```python
from build123d import *

# Parameters (mm, degrees)
SKETCH1_R                         = 60
BASE_BASE_DEPTH                   = 4
SIDE_START                        = -4
SIDE_CUTS_DEPTH                   = 4
SKETCH3_W                         = 5
SKETCH3_H                         = 13
TENDON_PASS_THROUGH_OPENING_DEPTH = 4
SKETCH4_R                         = 2.5
BASE_MOUNTING_HOLES_DEPTH         = 79.461200603
SKETCH5_W                         = 3
SKETCH5_H                         = 40
SKETCH5_W_2                       = 2.5
SKETCH5_H_2                       = 65
BOSS_EXTRUDE1_DEPTH               = 50
LPATTERN1_COUNT                   = 2
LPATTERN1_PITCH                   = 54
CUT_EXTRUDE1_REACH                = 138.279
SKETCH7_R                         = 3
CUT_EXTRUDE2_START                = -35
SKETCH9_R                         = 1
CUT_EXTRUDE2_DEPTH                = 35
LPATTERN2_COUNT                   = 2
LPATTERN2_PITCH                   = 96.6
FILLET1_R                         = 1
FILLET2_R                         = 1
SKETCH11_W                        = 12
SKETCH11_H                        = 6
CUT_EXTRUDE3_DEPTH                = 41
FILLET3_R                         = 1
FILLET4_R                         = 1
CUT_EXTRUDE4_REACH                = 104.781
SKETCH12_W                        = 20
SKETCH12_H                        = 8
FILLET5_R                         = 1


with BuildPart() as part:
    # Sketch1 → Base Base (new body)
    with BuildSketch(Plane(origin=(0, 0, 0), x_dir=(1, 0, 0), z_dir=(0, 1, 0))):
        with Locations(Location((0, 0, 0), (0, 0, 270))):
            Circle(SKETCH1_R)
    base_base = extrude(amount=BASE_BASE_DEPTH)

    # Sketch2 → Side Cuts (cut)
    with BuildSketch(Plane(origin=(0, 4, 0), x_dir=(1, 0, 0), z_dir=(0, 1, 0)).offset(SIDE_START)):
        with BuildLine():
            Line((-32.555183919, 50.4), (32.555183919, 50.4))
            ThreePointArc((32.555183919, 50.4), (0, 60), (-32.555183919, 50.4))
        make_face()
        with BuildLine():
            Line((-32.555183919, -50.4), (32.555183919, -50.4))
            ThreePointArc((32.555183919, -50.4), (0, -60), (-32.555183919, -50.4))
        make_face()
    extrude(amount=SIDE_CUTS_DEPTH, mode=Mode.SUBTRACT)

    # Sketch3 → Tendon Pass Through Opening (cut)
    with BuildSketch(Plane(origin=(0, 4, 0), x_dir=(1, 0, 0), z_dir=(0, 1, 0))):
        with Locations((32.5, 0)):
            Rectangle(SKETCH3_W, SKETCH3_H)
        with Locations((-32.5, 0)):
            Rectangle(SKETCH3_W, SKETCH3_H)
    extrude(amount=-TENDON_PASS_THROUGH_OPENING_DEPTH, mode=Mode.SUBTRACT)

    # Sketch4 → Base Mounting Holes (cut, through all)
    with BuildSketch(Plane(origin=(0, 4, 0), x_dir=(1, 0, 0), z_dir=(0, 1, 0))):
        with Locations(Location((32.5, 19, 0), (0, 0, 270))):
            Circle(SKETCH4_R)
        with Locations(Location((32.5, -19, 0), (0, 0, 90))):
            Circle(SKETCH4_R)
        with Locations(Location((-32.5, -19, 0), (0, 0, 270))):
            Circle(SKETCH4_R)
        with Locations(Location((-32.5, 19, 0), (0, 0, 90))):
            Circle(SKETCH4_R)
    extrude(amount=-BASE_MOUNTING_HOLES_DEPTH, mode=Mode.SUBTRACT)

    # Sketch5 → Boss-Extrude1 (add)
    with BuildSketch(Plane.XZ):
        with Locations((-48.3, -6)):
            Rectangle(SKETCH5_W, SKETCH5_H)
        with Locations((16.25, 11.5)):
            Rectangle(SKETCH5_W_2, SKETCH5_H_2)
        with Locations((48.3, -6)):
            Rectangle(SKETCH5_W, SKETCH5_H)
        with Locations((-16.25, 11.5)):
            Rectangle(SKETCH5_W_2, SKETCH5_H_2)
    extrude(amount=BOSS_EXTRUDE1_DEPTH)

    # LPattern1: Base Base ×2
    with Locations(*[(0, -i * LPATTERN1_PITCH, 0) for i in range(1, LPATTERN1_COUNT)]):
        add(base_base)

    # Sketch7 → Cut-Extrude1 (cut, up to next)
    with BuildSketch(Plane.ZY.offset(49.8), mode=Mode.PRIVATE) as cut_extrude1_sk1:
        with Locations((5.177676652, -18.760132428)):
            Circle(SKETCH7_R)
    cut_extrude1_tool1 = extrude(cut_extrude1_sk1.sketch, amount=-CUT_EXTRUDE1_REACH, mode=Mode.PRIVATE) & part.part
    # Sketch7 → Cut-Extrude1 (cut, up to next)
    with BuildSketch(Plane.ZY.offset(49.8), mode=Mode.PRIVATE) as cut_extrude1_sk2:
        with Locations((5.177676652, -42.760132428)):
            Circle(SKETCH7_R)
    cut_extrude1_tool2 = extrude(cut_extrude1_sk2.sketch, amount=-CUT_EXTRUDE1_REACH, mode=Mode.PRIVATE) & part.part
    cut_extrude1_1 = cut_extrude1_tool1.solids().sort_by_distance((-49.8, -18.760132, 5.177677))[0]
    add(cut_extrude1_1, mode=Mode.SUBTRACT)
    cut_extrude1_2 = cut_extrude1_tool2.solids().sort_by_distance((-49.8, -42.760132, 5.177677))[0]
    add(cut_extrude1_2, mode=Mode.SUBTRACT)
    cut_extrude1 = cut_extrude1_1 + cut_extrude1_2  # Cut-Extrude1 as one shape, for the pattern or mirror that repeats it

    # Sketch9 → Cut-Extrude2 (cut)
    with BuildSketch(Plane.ZY.offset(17.5).offset(CUT_EXTRUDE2_START)):
        with Locations((4.875, -18.760132428)):
            Circle(SKETCH9_R)
        with Locations((4.875, -42.760132428)):
            Circle(SKETCH9_R)
        with Locations((16.875, -18.760132428)):
            Circle(SKETCH9_R)
        with Locations((16.875, -42.760132428)):
            Circle(SKETCH9_R)
    extrude(amount=CUT_EXTRUDE2_DEPTH, mode=Mode.SUBTRACT)

    # LPattern2: Cut-Extrude1 ×2
    with Locations(*[(i * LPATTERN2_PITCH, 0, 0) for i in range(1, LPATTERN2_COUNT)]):
        add(cut_extrude1, mode=Mode.SUBTRACT)

    # Fillet1
    fillet1_edges = [part.edges().sort_by_distance(p)[0] for p in [
        (-30, 0, 0),
    ]]
    fillet(fillet1_edges, radius=FILLET1_R)

    # Fillet2
    fillet2_edges = [part.edges().sort_by_distance(p)[0] for p in [
        (30, 0, 0),
    ]]
    fillet(fillet2_edges, radius=FILLET2_R)

    # Sketch11 → Cut-Extrude3 (cut)
    with BuildSketch(Plane(origin=(17.5, 0, 0), x_dir=(0, 0, -1), z_dir=(1, 0, 0))):
        with Locations((-10.875, -5.611758363)):
            Rectangle(SKETCH11_W, SKETCH11_H)
    extrude(amount=-CUT_EXTRUDE3_DEPTH, mode=Mode.SUBTRACT)

    # Fillet3
    fillet3_edges = [part.edges().sort_by_distance(p)[0] for p in [
        (-17.5, -8.611758363, 10.875),
        (15, -8.611758363, 10.875),
        (-15, -8.611758363, 10.875),
        (17.5, -8.611758363, 10.875),
    ]]
    fillet(fillet3_edges, radius=FILLET3_R)

    # Fillet4
    fillet4_edges = [part.edges().sort_by_distance(p)[0] for p in [
        (-17.5, -6.111758363, 16.875),
        (15, -6.111758363, 16.875),
        (-15, -6.111758363, 16.875),
        (17.5, -6.111758363, 16.875),
        (-15, -6.111758363, 4.875),
        (-17.5, -6.111758363, 4.875),
        (17.5, -6.111758363, 4.875),
        (15, -6.111758363, 4.875),
    ]]
    fillet(fillet4_edges, radius=FILLET4_R - 0.0001)  # a hair under: the kernel refuses the full size

    # Sketch12 → Cut-Extrude4 (cut, up to next)
    with BuildSketch(Plane(origin=(0, 4, 0), x_dir=(1, 0, 0), z_dir=(0, 1, 0)), mode=Mode.PRIVATE) as cut_extrude4_sk1:
        Rectangle(SKETCH12_W, SKETCH12_H)
    cut_extrude4_tool1 = extrude(cut_extrude4_sk1.sketch, amount=-CUT_EXTRUDE4_REACH, mode=Mode.PRIVATE) & part.part
    add(cut_extrude4_tool1.solids().sort_by_distance((0, 4, 0))[0], mode=Mode.SUBTRACT)

    # Fillet5
    fillet5_edges = [part.edges().sort_by_distance(p)[0] for p in [
        (-10, 4, 0),
        (0, 4, 4),
        (10, 4, 0),
        (0, 4, -4),
        (0, 0, 4),
        (-10, 0, 0),
        (0, 0, -4),
        (10, 0, 0),
    ]]
    fillet(fillet5_edges, radius=FILLET5_R)


solid = part.part
```
The listing builds one solid part. Answer for the finished solid, in the listing's coordinates (mm). A direction names the side the tool comes from. Coordinates: 2 decimals unless noted, no trailing zeros. Loops run counter-clockwise (first coordinate to the right, second up) from the corner with the lowest first, then second, coordinate; pieces in that order, holes last. Notation, with made-up numbers: (70.5, 15.25) -> (103.5, 15.25) arc R12 cw to (103.5, 25.25) -> close; hole circle Ø10 at (75.25, 9.25). An arc over 180 degrees is marked (long way). Use one line per item in the form item = value. Start each with the question number.
Item 1: The part is cut by section D-D on z = -34.5. Determine the outline of the cut face in (x, y), then the cut area to 3 significant figures.
Item 2: The part is cut by section B-B on y = -48. Determine the outline of the cut face in (x, z).
Item 3: Flat-ended cylindrical pins translate along their axes: pin 1 Ø2 at (x, y) = (16.5, -15.5) entering from -Z; pin 2 Ø3 at (x, y) = (-32.5, 1) entering from +Z; pin 3 Ø1.6 at (y, z) = (2, 0) entering from -X. Find the tip coordinate at first contact, or state that the pin passes through.
Item 4: Consider L1, parallel to X at y = -9.5, z = -11; L2, parallel to X at y = -9.5, z = 24; L3, parallel to Y at x = 41.5, z = 6. Determine where each line is inside the solid, lowest interval first. Write a range as [from, to].
Item 5: The part is cut by section C-C on z = 30.5. Determine the outline of the cut face in (x, y), then the cut area to 3 significant figures.
Item 6: The mould has two halves that part along X. Classify faces 6 (the face through (1, 0, 10)), 7 (the face through (-31, 2, 17)), 8 (the face through (48, -25, -26)), 9 (the face through (59.994, 1.972, 0.838)): released by +X, released by -X, zero draft, split by the parting line, or undercut.
Item 7: The part is cut by section A-A on x = 0. Determine the outline of the cut face in (y, z).
Item 8: A tool of negligible diameter and unlimited length cuts with its end or side. For faces 1 (the face through (48, -25, 14)), 2 (the face through (-48, -25, 14)), 3 (the face through (15, -25, 11)), 4 (the face through (48.28, -40.23, 6.79)), 5 (the face through (34, 2, -21)), from which of +Z, -Z, +X, -X, +Y, -Y can it reach the whole face along a straight path? Write none if from no direction.
Answer key:
q1.outline = (-49.09, -54) -> (49.09, -54) -> (49.09, -50) -> (-49.09, -50) -> close; (-49.09, 0) -> (49.09, 0) -> (49.09, 4) -> (-49.09, 4) -> close
q1.area = 785 mm2
q2.outline = (-49.8, -26) -> (-46.8, -26) -> (-46.8, 14) -> (-49.8, 14) -> close; (-17.5, -21) -> (-15, -21) -> (-15, 44) -> (-17.5, 44) -> close; (15, -21) -> (17.5, -21) -> (17.5, 44) -> (15, 44) -> close; (46.8, -26) -> (49.8, -26) -> (49.8, 14) -> (46.8, 14) -> close
q3.pin_1 = -21
q3.pin_2 = 50.4
q3.pin_3 = -60
q4.L1 = [-49.8, -46.8], [-17.5, -15], [15, 17.5], [46.8, 49.8]
q4.L2 = [-17.5, -15], [15, 17.5]
q4.L3 = [-54, -50], [0, 4]
q5.outline = (-51.67, -54) -> (51.67, -54) -> (51.67, -50) -> (17.5, -50) -> (17.5, 0) -> (51.67, 0) -> (51.67, 4) -> (-51.67, 4) -> (-51.67, 0) -> (-17.5, 0) -> (-17.5, -50) -> (-51.67, -50) -> close; hole (-15, -50) -> (15, -50) -> (15, 0) -> (-15, 0) -> close
q5.area = 1,080 mm2
q6.face_6 = undercut
q6.face_7 = undercut
q6.face_8 = zero draft
q6.face_9 = released by +X
q7.outline = (-54, -60) -> (-50, -60) -> (-50, 60) -> (-54, 60) -> close; (0, -50.4) -> (4, -50.4) -> (4, -5) arc R1 ccw to (3, -4) -> (1, -4) arc R1 ccw to (0, -5) -> close; (0, 5) arc R1 ccw to (1, 4) -> (3, 4) arc R1 ccw to (4, 5) -> (4, 50.4) -> (0, 50.4) -> close
q8.face_1 = +Z, +X
q8.face_2 = +Z, -X
q8.face_3 = +Z, -Z
q8.face_4 = +X
q8.face_5 = +Y
